```python
from build123d import *

# Parameters (mm, degrees)
SKETCH2_W           = 80
SKETCH2_H           = 92
SKETCH2_R           = 1.6
SKETCH2_R_2         = 2.6
SKETCH2_R_3         = 12
SKETCH2_R_4         = 3.675
SKETCH2_W_2         = 3.760660172
SKETCH2_H_2         = 11
BOSS_EXTRUDE1_DEPTH = 3.125
FILLET1_R           = 20
FILLET2_R           = 20
FILLET4_R           = 5
FILLET5_R           = 7


with BuildPart() as part:
    # Sketch2 → Boss-Extrude1 (new body)
    with BuildSketch(Plane(origin=(0, 0, 0), x_dir=(1, 0, 0), z_dir=(0, 1, 0))):
        with Locations((40, 46)):
            Rectangle(SKETCH2_W, SKETCH2_H)
        with Locations((29.5, 5)):
            Circle(SKETCH2_R, mode=Mode.SUBTRACT)
        with Locations((29.5, 36)):
            Circle(SKETCH2_R, mode=Mode.SUBTRACT)
        with Locations((60.5, 36)):
            Circle(SKETCH2_R, mode=Mode.SUBTRACT)
        with Locations((60.5, 5)):
            Circle(SKETCH2_R, mode=Mode.SUBTRACT)
        with Locations((18, 45)):
            Circle(SKETCH2_R_2, mode=Mode.SUBTRACT)
        with Locations((72, 45)):
            Circle(SKETCH2_R_2, mode=Mode.SUBTRACT)
        with Locations((45, 20.5)):
            Circle(SKETCH2_R_3, mode=Mode.SUBTRACT)
        with Locations((45, 85)):
            Circle(SKETCH2_R_4, mode=Mode.SUBTRACT)
        with Locations((10, 53)):
            Circle(SKETCH2_R_2, mode=Mode.SUBTRACT)
        with Locations((10, 73)):
            Circle(SKETCH2_R_2, mode=Mode.SUBTRACT)
        with Locations((3.680330086, 73)):
            Rectangle(SKETCH2_W_2, SKETCH2_H_2, mode=Mode.SUBTRACT)
    extrude(amount=BOSS_EXTRUDE1_DEPTH)

    # Fillet1
    fillet1_edges = [part.edges().sort_by_distance(p)[0] for p in [
        (80, 1.5625, 0),
    ]]
    fillet(fillet1_edges, radius=FILLET1_R)

    # Fillet2
    fillet2_edges = [part.edges().sort_by_distance(p)[0] for p in [
        (0, 1.5625, 0),
    ]]
    fillet(fillet2_edges, radius=FILLET2_R)

    # Fillet4
    fillet4_edges = [part.edges().sort_by_distance(p)[0] for p in [
        (80, 1.5625, -92),
    ]]
    fillet(fillet4_edges, radius=FILLET4_R)

    # Fillet5
    fillet5_edges = [part.edges().sort_by_distance(p)[0] for p in [
        (0, 1.5625, -92),
    ]]
    fillet(fillet5_edges, radius=FILLET5_R)


solid = part.part
```
CAD build for the part. Positions are in the model's coordinates, mm. A direction names the side the tool comes from. Round coordinates to 2 decimals unless told otherwise and drop trailing zeros. Loops run counter-clockwise (first coordinate to the right, second up) from the corner with the lowest first, then second, coordinate; pieces in that order, holes last. Notation, with made-up numbers: M 75,23 L 95,23 A21 ccw 95,46 Z; hole C 36,8 d9. An arc over 180 degrees is marked long. Return JSON: item names as keys, results as strings. Group by question number.
(1) Drop flat-ended pins along their axis: P1, Ø1.5, axis at x = 13.5, y = 1, coming from the +Z side; P2, Ø1.6, axis at x = 3.5, y = 1.5, coming from the +Z side. Give the stop position or say it passes through.
(2) Saw through at C-C, the plane x = 18. List the corners of the cut face in (y, z) (3 decimals).
(3) Saw through at D-D, the plane y = 0.9. Give the number of separate pieces and of enclosed holes in the cut face, and give its area (3 significant figures).
(4) Saw through at A-A, the plane z = -53. List the corners of the cut face in (x, y) (3 decimals), and give its area (3 significant figures).
(5) Saw through at B-B, the plane z = -36. List the corners of the cut face in (x, y) (3 decimals).
(6) Tool access for faces 1 (the flat face through (41, 2, -92)), 2 (the flat face through (5.561, 2, -73)): list every direction of +Z, -Z, +X, -X, +Y, -Y with a clear straight run to the whole face (end or side of a thin tool).
(7) Wall check: probe 1 along X at (y, z) = (0.85, -36); probe 2 along Z at (x, y) = (45, 1.35) (3 decimals); probe 3 along X at (y, z) = (0.35, -76). Give the ranges that are in metal, low to high. Write a range as [from, to].
(8) Mould opens along Z. For faces 3 (the cylindrical face through (9.44, 1.54, -50.46)), 4 (the cylindrical face through (73.986, 1.584, -5.703)), 5 (the flat face through (39, 3.125, -47)) say: +Z half, -Z half, draft (parallel to the pull), parting line (faces both ways), or undercut.
Answer list:
{
 "1": {"P1": "z = -0.84", "P2": "z = -7.61"},
 "2": {"outline": "M 0,-92 L 3.125,-92 L 3.125,-47.6 L 0,-47.6 Z; M 0,-42.4 L 3.125,-42.4 L 3.125,-0.1 L 0,-0.1 Z"},
 "3": {"separate pieces": "1", "enclosed holes": "11", "area": "6,520 mm2"},
 "4": {"outline": "M 0,0 L 7.4,0 L 7.4,3.125 L 0,3.125 Z; M 12.6,0 L 80,0 L 80,3.125 L 12.6,3.125 Z", "area": "234 mm2"},
 "5": {"outline": "M 0,0 L 27.9,0 L 27.9,3.125 L 0,3.125 Z; M 31.1,0 L 58.9,0 L 58.9,3.125 L 31.1,3.125 Z; M 62.1,0 L 80,0 L 80,3.125 L 62.1,3.125 Z"},
 "6": {"face 1": "-Z, +X, -X, +Y, -Y", "face 2": "+Y, -Y"},
 "7": {"probe 1": "[0, 27.9], [31.1, 58.9], [62.1, 80]", "probe 2": "[-92, -88.675], [-81.325, -32.5], [-8.5, 0]", "probe 3": "[0, 1.8], [5.56, 80]"},
 "8": {"face 3": "undercut", "face 4": "+Z half", "face 5": "draft"}
}
